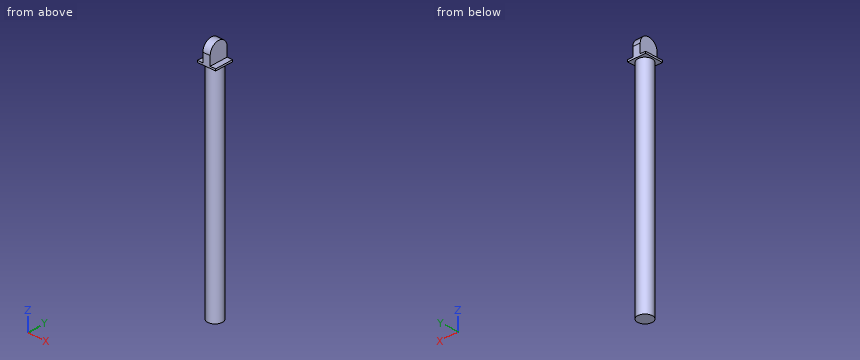
from build123d import *

# Parameters (mm, degrees)
SKETCH_1_W          = 10
SKETCH_1_H          = 10
EXTRUDE_1_DEPTH     = 11
SKETCH_2_W          = 3
SKETCH_2_H          = 10
CUT_EXTRUDE_1_DEPTH = 11
SKETCH_3_R          = 4
EXTRUDE_2_DEPTH     = 120
CUT_EXTRUDE_2_DEPTH = 80


with BuildPart() as part:
    # 草图1 → 凸台-拉伸1 (new body)
    with BuildSketch(Plane.XY):
        Rectangle(SKETCH_1_W, SKETCH_1_H)
    extrude(amount=EXTRUDE_1_DEPTH)

    # 草图2 → 切除-拉伸1 (cut)
    with BuildSketch(Plane(origin=(0, 5, 0), x_dir=(1, 0, 0), z_dir=(0, 1, 0))):
        with Locations((-3.5, -6)):
            Rectangle(SKETCH_2_W, SKETCH_2_H)
        with Locations((3.5, -6)):
            Rectangle(SKETCH_2_W, SKETCH_2_H)
    extrude(amount=-CUT_EXTRUDE_1_DEPTH, mode=Mode.SUBTRACT)

    # 草图3 → 凸台-拉伸2 (add)
    with BuildSketch(Plane(origin=(0, 0, 0), x_dir=(-1, 0, 0), z_dir=(0, 0, -1))):
        Circle(SKETCH_3_R)
    extrude(amount=EXTRUDE_2_DEPTH)

    # 草图4 → 切除-拉伸2 (cut)
    with BuildSketch(Plane(origin=(2, 0, 0), x_dir=(0, 0, -1), z_dir=(1, 0, 0))):
        with BuildLine():
            Line((-6, 5), (-12.295699944, 5))
            Line((-12.295699944, 5), (-12.295699944, -5))
            Line((-12.295699944, -5), (-6, -5))
            ThreePointArc((-6, -5), (-11, 0), (-6, 5))
        make_face()
    extrude(amount=-CUT_EXTRUDE_2_DEPTH, mode=Mode.SUBTRACT)


solid = part.part
Check sheet for the modelled part. Datum: model origin and axes. Units: mm. Coordinates: 2 decimals unless noted, no trailing zeros. Write each loop counter-clockwise with the first axis right and the second up, starting at its lowest first coordinate (ties: lowest second). Pieces come first, ordered by that corner, then holes. Notation, with made-up numbers: M -29,-3.5 L -6,-3.5 A9 ccw -6,2.5 Z; hole C -19.75,5.5 d7. An arc over 180 degrees is marked long. Answer as CSV lines item,"result".
Q1. Cross-section at B-B (x = 0). Record the boundary of the cut face in (y, z).
Check result:
outline,"M -5,0 L -4,0 L -4,-120 L 4,-120 L 4,0 L 5,0 L 5,6 A5 ccw -5,6 Z"
Q2. Cross-section at A-A (y = 0). Record the boundary of the cut face in (x, z), then the cut area to 3 significant figures.
Check result:
outline,"M -5,0 L -4,0 L -4,-120 L 4,-120 L 4,0 L 5,0 L 5,1 L 2,1 L 2,11 L -2,11 L -2,1 L -5,1 Z"
area,"1,010 mm^2"
Q3. Material ranges on probe 1 along Z at (x, y) = (-4.25, 0); probe 2 along Y at (x, z) = (-0.25, -109); probe 3 along Z at (x, y) = (-3.5, -1), recorded low to high. Write a range as from..to.
Check result:
probe 1,"0..1"
probe 2,"-3.99..3.99"
probe 3,"-120..1"
Q4. Cross-section at C-C (z = -62). Record the boundary of the cut face in (x, y), then the cut area to 3 significant figures.
Check result:
outline,"C 0,0 d8"
area,"50.3 mm^2"
Q5. Go/stop test with flat-tipped pins: pin 1 (5 mm diameter, centred on y = -2, z = -54.5, fed in from -X); pin 2 (3 mm diameter, centred on y = 2.5, z = 3.5, fed in from -X); pin 3 (1.5 mm diameter, centred on y = -1.5, z = -85.5, fed in from -X). Record where each tip stops, or that it passes through.
Check result:
pin 1,"x = -4"
pin 2,"x = -2"
pin 3,"x = -3.93"
